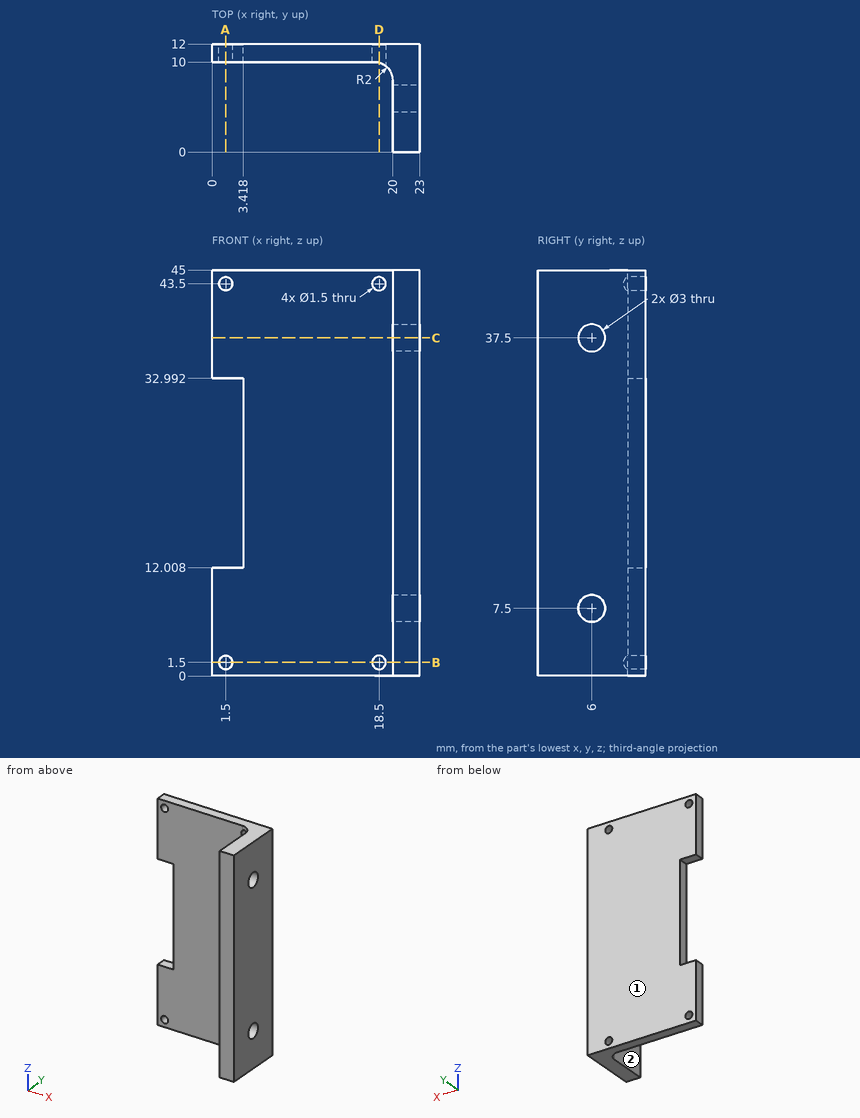
Check sheet for the drawn part. Datum: minimum x, y, z corner. Units: mm. A direction names the side the tool comes from. Round coordinates to 2 decimals unless told otherwise and drop trailing zeros. Write each loop counter-clockwise with the first axis right and the second up, starting at its lowest first coordinate (ties: lowest second). Pieces come first, ordered by that corner, then holes. Notation, with made-up numbers: (-3.5, -34) -> (12.5, -34) arc R18 ccw to (12.5, -17) -> close; hole circle Ø7 at (17.5, 25.5). An arc over 180 degrees is marked (long way). Write each question's results on one line, items separated by ' | '. Start each with the question number.
1. Cross-section at B-B (z = 1.5). Enter the section's corners in (x, y).
2. Cross-section at A-A (x = 1.5). Enter the section's corners in (y, z).
3. Depth check by flat-ended pin: P1, Ø2, axis at y = 11, z = 22, coming from the -X side; P2, Ø2.5, axis at y = 5.5, z = 20, coming from the -X side; P3, Ø2, axis at x = 1.5, z = 43.5, coming from the -Y side. Enter the tip coordinate at first touch or a pass-through.
4. Material ranges on probe 1 along Z at (x, y) = (1.5, 10.45); probe 2 along Z at (x, y) = (18.5, 10.9); probe 3 along X at (y, z) = (5.75, 24), recorded low to high. Write a range as from..to.
5. Cross-section at C-C (z = 37.5). Enter the section's corners in (x, y).
6. Cross-section at D-D (x = 18.5). Enter the section's corners in (y, z).
7. Set-up check for the marked faces 1 and 2: record each of +Z, -Z, +X, -X, +Y, -Y from which the full face is reachable in a straight line by a thin tool's end or side.
Solutions:
1) outline: (0, 10) -> (0.75, 10) -> (0.75, 12) -> (0, 12) -> close; (2.25, 10) -> (17.75, 10) -> (17.75, 12) -> (2.25, 12) -> close; (19.25, 9.56) arc R2 cw to (20, 8) -> (20, 0) -> (23, 0) -> (23, 12) -> (19.25, 12) -> close
2) outline: (10, 0) -> (12, 0) -> (12, 0.75) -> (10, 0.75) -> close; (10, 2.25) -> (12, 2.25) -> (12, 12.01) -> (10, 12.01) -> close; (10, 32.99) -> (12, 32.99) -> (12, 42.75) -> (10, 42.75) -> close; (10, 44.25) -> (12, 44.25) -> (12, 45) -> (10, 45) -> close
3) P1: stops at x = 3.42 | P2: stops at x = 20 | P3: stops at y = 10
4) probe 1: z = 0..0.75, 2.25..12.01, 32.99..42.75, 44.25..45 | probe 2: z = 0..0.75, 2.25..42.75, 44.25..45 | probe 3: x = 20..23
5) outline: (0, 10) -> (18, 10) arc R2 cw to (20, 8) -> (20, 7.5) -> (23, 7.5) -> (23, 12) -> (0, 12) -> close; (20, 0) -> (23, 0) -> (23, 4.5) -> (20, 4.5) -> close
6) outline: (9.94, 0) -> (12, 0) -> (12, 0.75) -> (9.94, 0.75) -> close; (9.94, 2.25) -> (12, 2.25) -> (12, 42.75) -> (9.94, 42.75) -> close; (9.94, 44.25) -> (12, 44.25) -> (12, 45) -> (9.94, 45) -> close
7) face 1: +Z, -Z, +X, -X, +Y | face 2: +Z, -Z, -X, -Y
